The drawing under review shows one solid part. Ordinate dimensions are in mm from its lowest x, y, z. Round coordinates to 2 decimals unless told otherwise and drop trailing zeros. Order: outer loops, then holes, each group sorted by start corner. A loop starts at its lowest first (then second) coordinate and runs counter-clockwise, first axis right, second up. Notation, with made-up numbers: (-18.5, 0) -> (19.5, 0) arc R12 ccw to (19.5, 7) -> close; hole circle Ø7 at (25.5, -21). An arc over 180 degrees is marked (long way). Return JSON: item names as keys, results as strings. Group by question number.
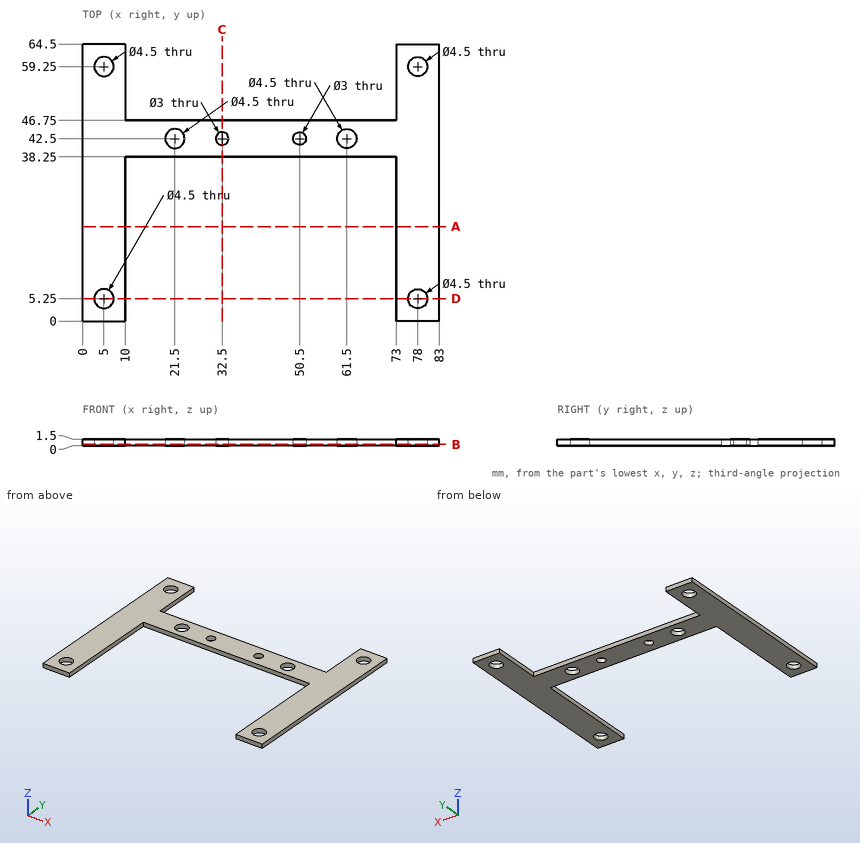
Item 1: Consider section B-B on z = 0.3. Give the number of separate pieces and of enclosed holes in the cut face, plus the area to 3 significant figures.
Item 2: Consider section A-A on y = 22. State the section outline as (x, z) points, plus the area to 3 significant figures.
Item 3: Consider section C-C on x = 32.5. State the section outline as (y, z) points, plus the area to 3 significant figures.
Item 4: Consider section D-D on y = 5.25. State the section outline as (x, z) points, plus the area to 3 significant figures.
Item 5: Insertion check: pin 1 Ø5 at (x, y) = (61.5, 42.5) entering from -Z. The pin has a flat end and moves straight along its axis. Give the tip position at first contact, or say it passes through.
Item 6: Wall thickness on line 1 along Y through (x, z) = (78, 0.6); line 2 along X through (y, z) = (59.5, 0.5); line 3 along Y through (x, z) = (32.5, 0.5): over which ranges is each line inside the solid? List them lowest first.
Values:
{
 "1": {"separate pieces": "1", "enclosed holes": "8", "area": "1,720 mm^2"},
 "2": {"outline": "(0, 0) -> (10, 0) -> (10, 1.5) -> (0, 1.5) -> close; (73, 0) -> (83, 0) -> (83, 1.5) -> (73, 1.5) -> close", "area": "30.0 mm^2"},
 "3": {"outline": "(38.25, 0) -> (41, 0) -> (41, 1.5) -> (38.25, 1.5) -> close; (44, 0) -> (46.75, 0) -> (46.75, 1.5) -> (44, 1.5) -> close", "area": "8.25 mm^2"},
 "4": {"outline": "(0, 0) -> (2.75, 0) -> (2.75, 1.5) -> (0, 1.5) -> close; (7.25, 0) -> (10, 0) -> (10, 1.5) -> (7.25, 1.5) -> close; (73, 0) -> (75.75, 0) -> (75.75, 1.5) -> (73, 1.5) -> close; (80.25, 0) -> (83, 0) -> (83, 1.5) -> (80.25, 1.5) -> close", "area": "16.5 mm^2"},
 "5": {"pin 1": "z = 0"},
 "6": {"line 1": "0 to 3, 7.5 to 57, 61.5 to 64.5", "line 2": "0 to 2.76, 7.24 to 10, 73 to 75.76, 80.24 to 83", "line 3": "38.25 to 41, 44 to 46.75"}
}
